For this review, take the finished solid that the model builds, in its own axes (mm). Coordinates: 2 decimals unless noted, no trailing zeros. Loops run counter-clockwise (first coordinate to the right, second up) from the corner with the lowest first, then second, coordinate; pieces in that order, holes last. Notation, with made-up numbers: M 56,-34 L 70,-34 A12 cw 70,-28 Z; hole C -5,-2.75 d5. An arc over 180 degrees is marked long. Use one line per item in the form item = value.
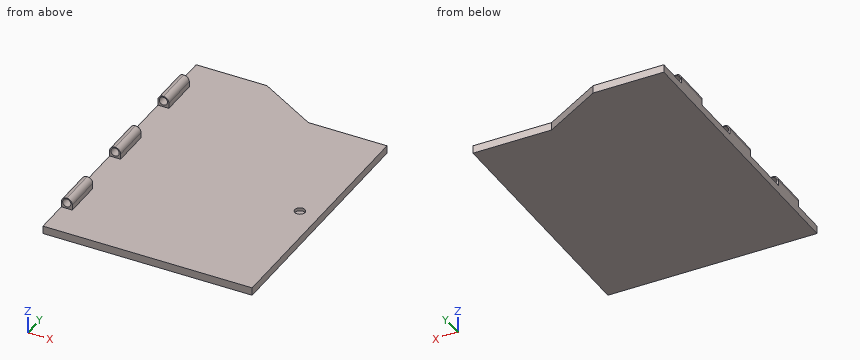
```python
from build123d import *

# Parameters (mm, degrees)
F0_W     = 7
F0_H     = 24.5
F1_DEPTH = 5
F2_W     = 7
F2_H     = 24.5
F3_DEPTH = 7
F4_R     = 3.49999
F5_R     = 2.625
F6_DEPTH = 162.001
F7_R     = 3.25
F8_DEPTH = 2


# Not quite as in the source:
# - a fillet or chamfer is up to 0.001 mm smaller than in the source, because OpenCascade refuses the exact size


with BuildPart() as f1:
    # F0 (on Top) → F1 (new body)
    with BuildSketch(Plane.XY):
        Polygon((-34.0007612563, 142.7090217992), (-79.0007612563, 142.7090217992), (-79.0007612563, 121.2090217992), (-72.0007612563, 121.2090217992), (-72.0007612563, 96.7090217992), (-79.0007612563, 96.7090217992), (-79.0007612563, 63.2090217992), (-72.0007612563, 63.2090217992), (-72.0007612563, 38.7090217992), (-79.0007612563, 38.7090217992), (-79.0007612563, 5.2090217992), (-72.0007612563, 5.2090217992), (-72.0007612563, -19.2909782008), (-79.0007612563, -19.2909782008), (-79.0007612563, -41.2909782008), (53.9992387437, -41.2909782008), (53.9992387437, 120.7090218186), (3.9992387437, 120.7090218186), align=None)
        with Locations((-75.5007612563, 108.9590217992)):
            Rectangle(F0_W, F0_H)
        with Locations((-75.5007612563, 50.9590217992)):
            Rectangle(F0_W, F0_H)
        with Locations((-75.5007612563, -7.0409782008)):
            Rectangle(F0_W, F0_H)
    extrude(amount=F1_DEPTH)

    # F2 (on face) → F3 (join)
    with BuildSketch(Plane.XY.offset(5)):
        with Locations((-75.5007612563, 108.9590217992)):
            Rectangle(F2_W, F2_H)
        with Locations((-75.5007612563, 50.9590217992)):
            Rectangle(F2_W, F2_H)
        with Locations((-75.5007612563, -7.0409782008)):
            Rectangle(F2_W, F2_H)
    extrude(amount=F3_DEPTH)

    # F4 (radius 3.5 in the source; OpenCascade refuses exactly that, so slightly less here)
    f4_edges = [f1.edges().sort_by_distance(p)[0] for p in [
        (-72.000761, 108.959022, 12),
        (-72.000761, 50.959022, 12),
        (-79.000761, 50.959022, 12),
        (-79.000761, 108.959022, 12),
        (-72.000761, -7.040978, 12),
        (-79.000761, -7.040978, 12),
    ]]
    fillet(f4_edges, radius=F4_R)

    # F5 (on face) → F6 (cut, through all)
    with BuildSketch(Plane.XZ.offset(19.2909782008)):
        with Locations((-75.5007612563, 8.75)):
            Circle(F5_R)
    extrude(amount=-F6_DEPTH, mode=Mode.SUBTRACT)

    # F7 (on face) → F8 (cut)
    with BuildSketch(Plane.XY.offset(5)):
        with Locations((41.4992387437, 39.7090218089)):
            Circle(F7_R)
    extrude(amount=-F8_DEPTH, mode=Mode.SUBTRACT)


solid = f1.part
```
1. Wall thickness on line 1 along Y through (x, z) = (37.5, 2); line 2 along Z through (x, y) = (-36.5, -21.5); line 3 along X through (y, z) = (-4.5, 5.5): over which ranges is each line inside the solid? List them lowest first. Write a range as from..to.
Computed values:
line_1 = -41.29..120.71
line_2 = 0..5
line_3 = -79..-72
2. For pin 1 Ø3 at (x, z) = (-75.5, 8.75) entering from -Y; pin 2 Ø1.1 at (y, z) = (-12, 7.5) entering from +X; pin 3 Ø5.5 at (x, z) = (-75.5, 8.5) entering from +Y; pin 4 Ø5.5 at (x, z) = (-76, 8.5) entering from -Y, all flat-tipped, find the tip position at first contact; note any pin that passes through.
Computed values:
pin_1 = through
pin_2 = -72
pin_3 = 121.21
pin_4 = -19.29
3. Consider section B-B on x = 21. Write out the cut boundary in (y, z).
Computed values:
outline = M -41.29,0 L 120.71,0 L 120.71,5 L -41.29,5 Z
4. Consider section C-C on y = 83. Write out the cut boundary in (x, z), plus the area to 3 significant figures.
Computed values:
outline = M -79,0 L 54,0 L 54,5 L -79,5 Z
area = 665 mm2
